from build123d import *

# Parameters (mm, degrees)
F0_W      = 215.9
F0_H      = 127
F1_DEPTH  = 25.4
F3_DEPTH  = 25.4
F4_DEPTH  = 25.4
F5_DEPTH  = 25.4
F6_DEPTH  = 25.4
F7_W      = 76.2
F7_H      = 76.2
F8_DEPTH  = 25.4
F9_W      = 19.05
F9_H      = 50.8
F10_DEPTH = 25.4


with BuildPart() as f1:
    # F0 (on Front) → F1 (new body)
    with BuildSketch(Plane.XZ):
        with Locations((12.806937, -5.306549)):
            Rectangle(F0_W, F0_H)
    extrude(amount=F1_DEPTH)

    # F2 (on face) → F3 (cut)
    with BuildSketch(Plane.XZ.offset(25.4)):
        Polygon((-95.143063, 58.193451), (-95.143063, 31.784684), (-44.460724, 58.193451), align=None)
    extrude(amount=-F3_DEPTH, mode=Mode.SUBTRACT)

    # F2 (on face) → F4 (cut)
    with BuildSketch(Plane.XZ.offset(25.4)):
        Polygon((-45.112216, -68.806549), (-95.143063, -41.183426), (-95.143063, -68.806549), align=None)
    extrude(amount=-F4_DEPTH, mode=Mode.SUBTRACT)

    # F2 (on face) → F5 (cut)
    with BuildSketch(Plane.XZ.offset(25.4)):
        Polygon((120.756937, -42.098548), (70.231644, -68.806549), (120.756937, -68.806549), align=None)
    extrude(amount=-F5_DEPTH, mode=Mode.SUBTRACT)

    # F2 (on face) → F6 (cut)
    with BuildSketch(Plane.XZ.offset(25.4)):
        Polygon((120.756937, 58.193451), (70.074598, 58.193451), (120.756937, 31.784684), align=None)
    extrude(amount=-F6_DEPTH, mode=Mode.SUBTRACT)

    # F7 (on face) → F8 (cut)
    with BuildSketch(Plane.XZ.offset(25.4)):
        with Locations((12.806937, -7.448901)):
            Rectangle(F7_W, F7_H)
    extrude(amount=-F8_DEPTH, mode=Mode.SUBTRACT)

    # F9 (on face) → F10 (cut)
    with BuildSketch(Plane.XZ.offset(25.4)):
        with Locations((-53.868063, -3.692623)):
            Rectangle(F9_W, F9_H)
        with Locations((79.481937, -3.208301)):
            Rectangle(F9_W, F9_H)
    extrude(amount=-F10_DEPTH, mode=Mode.SUBTRACT)


solid = f1.part
Here's how the part is built. I have some questions about the finished solid (model axes, mm). A direction names the side the tool comes from. Coordinates: 2 decimals unless noted, no trailing zeros. Loops run counter-clockwise (first coordinate to the right, second up) from the corner with the lowest first, then second, coordinate; pieces in that order, holes last.
1. Imagine slicing it at B-B, the plane z = -2. Please give me the cut outline in (x, y), and give its area (3 significant figures).
2. For P1, Ø15, axis at x = -58, y = -8.5, coming from the +Z side; P2, Ø9.5, axis at x = 83, y = -18, coming from the -Z side; P3, Ø15, axis at x = -56, y = -15.5, coming from the -Z side, each with a flat end and sliding along its axis, tell me the tip position at first contact or that it passes through.
3. Imagine slicing it at D-D, the plane y = -8. Please give me the cut outline in (x, z).
4. Imagine slicing it at A-A, the plane x = -13.5. Please give me the cut outline in (y, z).
5. For faces 4 (the flat face through (-69.777, -12.878, -55.188)), 5 (the flat face through (79, -13, -28.608)), which set-ups out of +Z, -Z, +X, -X, +Y, -Y let a thin tool reach every point of the face, with its end or its side?
6. I need wall thicknesses on L1, parallel to X at y = -11.75, z = -6; L2, parallel to Z at x = 8, y = -19.75; L3, parallel to X at y = -7.75, z = 25. Which ranges of each line are inside material? Lowest first, please.
7. Imagine slicing it at C-C, the plane z = -37. Please give me the cut outline in (x, y).
8. If we mould it in two halves opening along Z, with no side actions, what happens to faces 1 (the flat face through (11, 0, -47)), 2 (the flat face through (12, -13, 30.651)), 3 (the flat face through (12, -13, -68.807))? For each: pulls with the +Z half, pulls with the -Z half, needs draft (parallel to the pull), parting line crosses it, or undercut.
Taken from the geometry:
1. outline: (-95.14, -25.4) - (-63.39, -25.4) - (-63.39, 0) - (-95.14, 0) - close; (-44.34, -25.4) - (-25.29, -25.4) - (-25.29, 0) - (-44.34, 0) - close; (50.91, -25.4) - (69.96, -25.4) - (69.96, 0) - (50.91, 0) - close; (89.01, -25.4) - (120.76, -25.4) - (120.76, 0) - (89.01, 0) - close
1. area: 2,580 mm2
2. P1: stops at z = 55.05
2. P2: stops at z = -64.57
2. P3: stops at z = -66.94
3. outline: (-95.14, -41.18) - (-45.11, -68.81) - (70.23, -68.81) - (120.76, -42.1) - (120.76, 31.78) - (70.07, 58.19) - (-44.46, 58.19) - (-95.14, 31.78) - close; hole (-63.39, -29.09) - (-44.34, -29.09) - (-44.34, 21.71) - (-63.39, 21.71) - close; hole (-25.29, -45.55) - (50.91, -45.55) - (50.91, 30.65) - (-25.29, 30.65) - close; hole (69.96, -28.61) - (89.01, -28.61) - (89.01, 22.19) - (69.96, 22.19) - close
4. outline: (-25.4, -68.81) - (0, -68.81) - (0, -45.55) - (-25.4, -45.55) - close; (-25.4, 30.65) - (0, 30.65) - (0, 58.19) - (-25.4, 58.19) - close
5. face 4: -Z, -X, +Y, -Y
5. face 5: +Y, -Y
6. L1: x = -95.14 to -63.39, -44.34 to -25.29, 50.91 to 69.96, 89.01 to 120.76
6. L2: z = -68.81 to -45.55, 30.65 to 58.19
6. L3: x = -95.14 to -25.29, 50.91 to 120.76
7. outline: (-95.14, -25.4) - (-25.29, -25.4) - (-25.29, 0) - (-95.14, 0) - close; (50.91, -25.4) - (120.76, -25.4) - (120.76, 0) - (50.91, 0) - close
8. face 1: needs draft
8. face 2: undercut
8. face 3: pulls with the -Z half
